```python
from build123d import *

# Parameters (mm, degrees)
BOSS_EXTRUDE2_DEPTH = 64
SKETCH3_W           = 28
SKETCH3_H           = 44
CUT_EXTRUDE3_DEPTH  = 26
CUT_EXTRUDE4_DEPTH  = 82.510735489
CUT_EXTRUDE6_DEPTH  = 86.276022421


with BuildPart() as part:
    # Sketch1 → Boss-Extrude2 (new body)
    with BuildSketch(Plane.XY):
        Polygon((0, 0), (0, 42), (22, 42), (50, 16), (50, 0), (34, 0), (34, 6), (16, 6), (16, 0), align=None)
    extrude(amount=-BOSS_EXTRUDE2_DEPTH)

    # Sketch3 → Cut-Extrude3 (cut)
    with BuildSketch(Plane(origin=(0, 42, 0), x_dir=(1, 0, 0), z_dir=(0, 1, 0))):
        with Locations((36, 32)):
            Rectangle(SKETCH3_W, SKETCH3_H)
    extrude(amount=-CUT_EXTRUDE3_DEPTH, mode=Mode.SUBTRACT)

    # Sketch5 → Cut-Extrude4 (cut, through all)
    with BuildSketch(Plane(origin=(22, 0, 0), x_dir=(0, 0, -1), z_dir=(1, 0, 0))):
        Polygon((32, 27), (47, 42), (17, 42), align=None)
    extrude(amount=-CUT_EXTRUDE4_DEPTH, mode=Mode.SUBTRACT)

    # Sketch7 → Cut-Extrude6 (cut, through all)
    with BuildSketch(Plane(origin=(0, 16, 0), x_dir=(1, 0, 0), z_dir=(0, 1, 0))):
        Polygon((40, 32), (50, 41), (50, 23), align=None)
    extrude(amount=-CUT_EXTRUDE6_DEPTH, mode=Mode.SUBTRACT)


solid = part.part
```
Can you work these out from the model? Positions are in its coordinate system, mm. A direction names the side the tool comes from. Coordinates: 2 decimals unless noted, no trailing zeros. Loops run counter-clockwise (first coordinate to the right, second up) from the corner with the lowest first, then second, coordinate; pieces in that order, holes last. Notation, with made-up numbers: M 18.5,81.5 L 29.5,81.5 A29 ccw 29.5,110.5 Z; hole C 48,22.5 d7. An arc over 180 degrees is marked long. Put each result on its own line as item: value. Start each with the question number.
(1) Will these pins go through, and if not, where does the flat tip stop? pin 1 Ø1 at (y, z) = (33.5, -52.5) entering from +X; pin 2 Ø22.5 at (x, z) = (38, -31) entering from +Y; pin 3 Ø2 at (x, z) = (29.5, -47.5) entering from -Y.
(2) Imagine slicing it at D-D on y = 34. List the corners of the cut face in (x, z) for me, and give its area (3 significant figures).
(3) Imagine slicing it at B-B on x = 17. List the corners of the cut face in (y, z) for me.
(4) I need wall thicknesses on probe 1 along X at (y, z) = (2.5, -6); probe 2 along Z at (x, y) = (28, 29.5); probe 3 along Y at (x, z) = (45.5, -45.5). Which ranges of each line are inside material? Lowest first, please.
(5) Which directions (+Z, -Z, +X, -X, +Y, -Y) give clear straight access to the entire face, cutting with the end or side of a thin tool? Please do faces 5 (the face through (11, 34, -39)), 6 (the face through (16, 3, -32)), 7 (the face through (30, 23, -10)).
(6) Imagine slicing it at C-C on y = 7. List the corners of the cut face in (x, z) for me.
(7) We'd pull the mould along X, two halves only. Please class faces 1 (the face through (36, 29, -5)), 2 (the face through (34, 3, -32)), 3 (the face through (11, 35, -24)), 4 (the face through (25, 6, -32)): +X half, -X half, draft (parallel to the pull), parting line (faces both ways), or undercut.
(8) Imagine slicing it at A-A on z = -8.5. List the corners of the cut face in (x, y) for me.
Worked answers:
1. pin 1: stops at x = 22
1. pin 2: stops at y = 16
1. pin 3: stops at y = 6
2. outline: M 0,-64 L 30.62,-64 L 30.62,-54 L 22,-54 L 22,-39 L 0,-39 Z; M 0,-25 L 22,-25 L 22,-10 L 30.62,-10 L 30.62,0 L 0,0 Z
2. area: 1,270 mm2
3. outline: M 6,-64 L 42,-64 L 42,-47 L 27,-32 L 42,-17 L 42,0 L 6,0 Z
4. probe 1: x = 0 to 16, 34 to 50
4. probe 2: z = -64 to -54, -10 to 0
4. probe 3: y = 0 to 16
5. face 5: +X, -X, +Y
5. face 6: +Z, -Z, -Y
5. face 7: +X, +Y
6. outline: M 0,-64 L 50,-64 L 50,-41 L 40,-32 L 50,-23 L 50,0 L 0,0 Z
7. face 1: +X half
7. face 2: undercut
7. face 3: draft
7. face 4: undercut
8. outline: M 0,0 L 16,0 L 16,6 L 34,6 L 34,0 L 50,0 L 50,16 L 22,42 L 0,42 Z
